Check sheet for the modelled part. Datum: model origin and axes. Units: mm. Give positions to 0.01 mm unless a question says otherwise; leave off trailing zeros. Order: outer loops, then holes, each group sorted by start corner. A loop starts at its lowest first (then second) coordinate and runs counter-clockwise, first axis right, second up. Notation, with made-up numbers: (73.25, 81.25) -> (124.25, 81.25) arc R19 ccw to (124.25, 96.25) -> close; hole circle Ø1 at (0.5, 89). An arc over 180 degrees is marked (long way). Answer in a Markdown table with one row per item. Add a question column.
(1) Thickness scan on L1, parallel to Z at x = 0, y = 0.65; L2, parallel to X at y = 1.25, z = 69; L3, parallel to X at y = 0.2, z = 113. Record the ranges inside material, lowest first. Write a range as [from, to].
(2) Cross-section at A-A (x = 0). Record the cut outline in (y, z).
(3) Cross-section at B-B (z = 63). Record the cut outline in (x, y), then the cut area to 3 significant figures.
```python
from build123d import *

# Parameters (mm, degrees)
PAD_DEPTH       = 126
POCKET_DEPTH    = 5.801
FILLET_R        = 1
FILLET001_R     = 1
SKETCH002_R     = 1.7
POCKET001_DEPTH = 5


with BuildPart() as part:
    # Sketch → Pad (new body)
    with BuildSketch(Plane.XY):
        Polygon((-2.9, 0), (2.9, 0), (2.9, 2.4), (2.1, 2.4), (2.1, 0.8), (-2.1, 0.8), (-2.1, 2.4), (-2.9, 2.4), align=None)
    extrude(amount=PAD_DEPTH)

    # Sketch001 → Pocket (cut, through all)
    with BuildSketch(Plane.YZ.offset(2.9)):
        Polygon((0.8, 0), (0.8, 0.5), (2.4, 1), (2.4, 0), align=None)
        Polygon((0.8, 126), (2.4, 126), (2.4, 125), (0.8, 125.5), align=None)
    extrude(amount=-POCKET_DEPTH, mode=Mode.SUBTRACT)

    # Fillet
    fillet_edges = [part.edges().sort_by_distance(p)[0] for p in [
        (2.9, 0.4, 126),
        (-2.9, 0.4, 126),
        (2.9, 0.4, 0),
        (-2.9, 0.4, 0),
    ]]
    fillet(fillet_edges, radius=FILLET_R)

    # Fillet001
    fillet001_edges = [part.edges().sort_by_distance(p)[0] for p in [
        (2.5, 2.4, 1),
        (-2.5, 2.4, 1),
        (2.5, 2.4, 125),
        (-2.5, 2.4, 125),
    ]]
    fillet(fillet001_edges, radius=FILLET001_R)

    # Sketch002 → Pocket001 (cut)
    with BuildSketch(Plane.XZ):
        with Locations((0, 63)):
            Circle(SKETCH002_R)
        with Locations((0, 113)):
            Circle(SKETCH002_R)
        with Locations((0, 13)):
            Circle(SKETCH002_R)
    extrude(amount=-POCKET001_DEPTH, mode=Mode.SUBTRACT)


solid = part.part
```
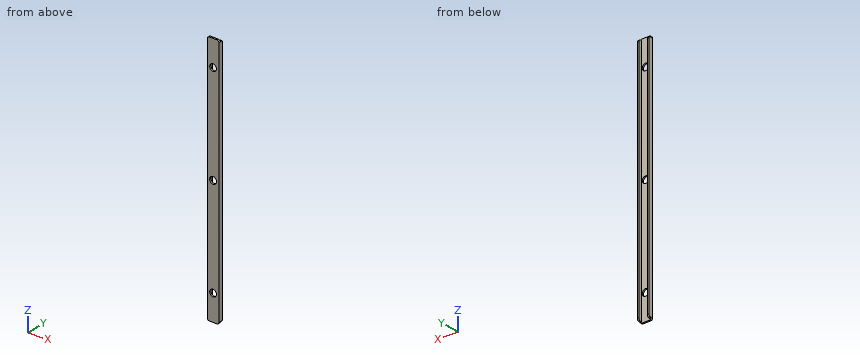
Answer below:
| question | item | result |
|---|---|---|
| 1 | L1 | z = [0, 11.3], [14.7, 61.3], [64.7, 111.3], [114.7, 126] |
| 1 | L2 | x = [-2.9, -2.1], [2.1, 2.9] |
| 1 | L3 | x = [-2.9, -1.7], [1.7, 2.9] |
| 2 | outline | (0, 0) -> (0.8, 0) -> (0.8, 11.3) -> (0, 11.3) -> close; (0, 14.7) -> (0.8, 14.7) -> (0.8, 61.3) -> (0, 61.3) -> close; (0, 64.7) -> (0.8, 64.7) -> (0.8, 111.3) -> (0, 111.3) -> close; (0, 114.7) -> (0.8, 114.7) -> (0.8, 126) -> (0, 126) -> close |
| 3 | outline | (-2.9, 0) -> (-1.7, 0) -> (-1.7, 0.8) -> (-2.1, 0.8) -> (-2.1, 2.4) -> (-2.9, 2.4) -> close; (1.7, 0) -> (2.9, 0) -> (2.9, 2.4) -> (2.1, 2.4) -> (2.1, 0.8) -> (1.7, 0.8) -> close |
| 3 | area | 4.48 mm² |
